CAD build for the part. Positions are in the model's coordinates, mm. Face numbers are marked on the shaded views. A direction names the side the tool comes from. Give positions to 0.01 mm unless a question says otherwise; leave off trailing zeros. Loops run counter-clockwise (first coordinate to the right, second up) from the corner with the lowest first, then second, coordinate; pieces in that order, holes last. Notation, with made-up numbers: (29.25, 79) -> (82.25, 79) arc R32 ccw to (82.25, 105) -> close; hole circle Ø10 at (6, 89). An arc over 180 degrees is marked (long way). Write each question's results on one line, items separated by ' | '. Start each with the question number.
```python
from build123d import *

# Parameters (mm, degrees)
EXTRUDE_1_DEPTH          = 21
SKETCH_2_R               = 7.5
EXTRUDE_2_DEPTH          = 2
SKETCH_3_R               = 9
EXTRUDE_3_DEPTH          = 3
SKETCH_4_R               = 10
EXTRUDE_4_DEPTH          = 8
SKETCH_5_R               = 7.5
EXTRUDE_5_DEPTH          = 2
CUT_EXTRUDE_1_DEPTH      = 42.106568818
CUT_EXTRUDE_1_DEPTH_BACK = 42.106568818
SKETCH_7_R               = 4
HOLE_WIZARD_G1_21_D      = 19
HOLE_WIZARD_G1_21_DEPTH  = 18
HOLE_WIZARD_G1_21_TIP    = 5.708175881
CHAMFER_1_SIZE           = 1
FILLET_1_R               = 1
SKETCH_10_R              = 5
CUT_EXTRUDE_2_DEPTH      = 40


with BuildPart() as part:
    # Эскиз1 → Бобышка-Вытянуть1 (new body)
    with BuildSketch(Plane(origin=(0, 0, 0), x_dir=(1, 0, 0), z_dir=(0, 1, 0))):
        Polygon((0, 15), (-12.990381057, 7.5), (-12.990381057, -7.5), (0, -15), (12.990381057, -7.5), (12.990381057, 7.5), align=None)
    extrude(amount=EXTRUDE_1_DEPTH)

    # Эскиз2 → Бобышка-Вытянуть2 (add)
    with BuildSketch(Plane(origin=(0, 21, 0), x_dir=(1, 0, 0), z_dir=(0, 1, 0))):
        with Locations(Location((0, 0, 0), (0, 0, 270))):
            Circle(SKETCH_2_R)
    extrude(amount=EXTRUDE_2_DEPTH)

    # Эскиз3 → Бобышка-Вытянуть3 (add)
    with BuildSketch(Plane(origin=(0, 23, 0), x_dir=(1, 0, 0), z_dir=(0, 1, 0))):
        with Locations(Location((0, 0, 0), (0, 0, 270))):
            Circle(SKETCH_3_R)
    extrude(amount=EXTRUDE_3_DEPTH)

    # Эскиз4 → Бобышка-Вытянуть4 (add)
    with BuildSketch(Plane(origin=(0, 26, 0), x_dir=(1, 0, 0), z_dir=(0, 1, 0))):
        with Locations(Location((0, 0, 0), (0, 0, 270))):
            Circle(SKETCH_4_R)
    extrude(amount=EXTRUDE_4_DEPTH)

    # Эскиз5 → Бобышка-Вытянуть5 (add)
    with BuildSketch(Plane(origin=(0, 34, 0), x_dir=(1, 0, 0), z_dir=(0, 1, 0))):
        with Locations(Location((0, 0, 0), (0, 0, 270))):
            Circle(SKETCH_5_R)
    extrude(amount=EXTRUDE_5_DEPTH)

    # Эскиз6 → Повернуть1 (revolve)
    with BuildSketch(Plane.XY, mode=Mode.PRIVATE) as revolve_1_sk:
        Polygon((-8, 37), (-6, 37), (-6, 36), (-4, 36), (-4, 38), (-8, 38), align=None)
    revolve(revolve_1_sk.sketch.rotate(Axis((0, 36, 0), (0, 1, 0)), 270), axis=Axis((0, 36, 0), (0, 1, 0)))

    # Эскиз7 → Вырез-Вытянуть1 (cut, two sides: drawn at the far end of the back side and taken through both)
    with BuildSketch(Plane(origin=(0, 36, 0), x_dir=(1, 0, 0), z_dir=(0, 1, 0)).offset(-CUT_EXTRUDE_1_DEPTH_BACK)):
        with Locations(Location((0, 0, 0), (0, 0, 90))):
            Circle(SKETCH_7_R)
    extrude(amount=CUT_EXTRUDE_1_DEPTH + CUT_EXTRUDE_1_DEPTH_BACK, mode=Mode.SUBTRACT)

    # Отверстие обработанное метчиком G1/21
    with Locations(Plane(origin=(0, 0, 0), x_dir=(-1, 0, 0), z_dir=(0, -1, 0))):
        with Locations((0, 0)):
            Hole(HOLE_WIZARD_G1_21_D / 2, depth=HOLE_WIZARD_G1_21_DEPTH)
            with Locations((0, 0, -(HOLE_WIZARD_G1_21_DEPTH + HOLE_WIZARD_G1_21_TIP / 2))):  # 118° drill point
                Cone(0, HOLE_WIZARD_G1_21_D / 2, HOLE_WIZARD_G1_21_TIP, mode=Mode.SUBTRACT)

    # Фаска1
    chamfer_1_edges = [part.edges().sort_by_distance(p)[0] for p in [
        (-12.990381057, 21, 0),
        (-6.495190528, 21, 11.25),
        (6.495190528, 21, 11.25),
        (12.990381057, 21, 0),
        (6.495190528, 21, -11.25),
        (-9.5, 0, 0),
        (12.990381057, 0, 0),
        (6.495190528, 0, 11.25),
        (-6.495190528, 0, 11.25),
        (-6.495190528, 21, -11.25),
        (-12.990381057, 0, 0),
        (-6.495190528, 0, -11.25),
        (6.495190528, 0, -11.25),
    ]]
    chamfer(chamfer_1_edges, length=CHAMFER_1_SIZE)

    # Скругление1
    fillet_1_edges = [part.edges().sort_by_distance(p)[0] for p in [
        (12.990381057, 10.5, -7.5),
        (12.990381057, 10.5, 7.5),
        (0, 10.5, 15),
        (-12.990381057, 10.5, 7.5),
        (-12.990381057, 10.5, -7.5),
        (0, 10.5, -15),
    ]]
    fillet(fillet_1_edges, radius=FILLET_1_R)

    # Эскиз10 → Вырез-Вытянуть2 (cut)
    with BuildSketch(Plane(origin=(0, 38, 0), x_dir=(1, 0, 0), z_dir=(0, 1, 0))):
        with Locations(Location((0, 0, 0), (0, 0, 270))):
            Circle(SKETCH_10_R)
    extrude(amount=-CUT_EXTRUDE_2_DEPTH, mode=Mode.SUBTRACT)


solid = part.part
```
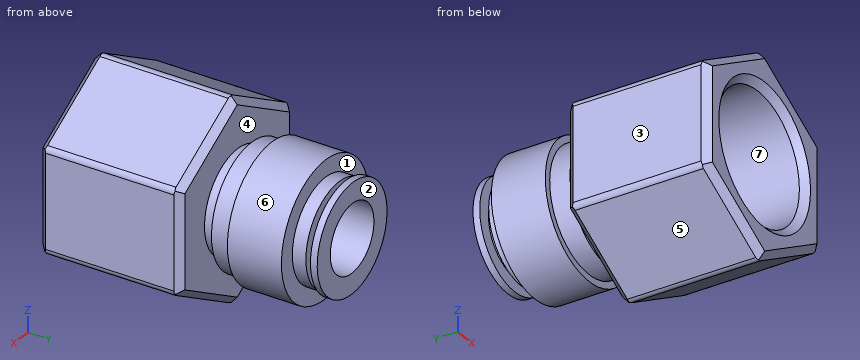
Q1. Saw through at A-A, the plane y = 5. List the corners of the cut face in (x, z).
Q2. Mould opens along Y. For the marked faces 1, 2 and 3 say: pulls with the +Y half, pulls with the -Y half, needs draft (parallel to the pull), parting line crosses it, or undercut.
Q3. Saw through at C-C, the plane x = 11.25. List the corners of the cut face in (y, z), then the cut area to 3 significant figures.
Q4. Drop flat-ended pins along their axis: pin 1 (5.5 mm diameter, centred on x = 3, z = -4, fed in from -Y); pin 2 (6 mm diameter, centred on x = 0, z = 0, fed in from -Y); pin 3 (5 mm diameter, centred on x = -2.5, z = 1.5, fed in from -Y); pin 4 (1.5 mm diameter, centred on x = -6.5, z = 0.5, fed in from -Y). Give the stop position or say it passes through.
Q5. Saw through at B-B, the plane z = 12. List the corners of the cut face in (x, y).
Q6. Saw through at D-D, the plane y = 33.5. List the corners of the cut face in (x, z).
Q7. Which spindle directions (+Z, -Z, +X, -X, +Y, -Y) get a long thin tool onto all of the face, cutting with end or side? Do the marked faces 4, 5, 6 and 7. Say none if no direction does.
Q8. Wall check: L1, parallel to Z at x = 0, y = 11.5; L2, parallel to X at y = 14.5, z = 0; L3, parallel to X at y = 30.5, z = 0. Give the ranges that are in metal, low to high.
Answer block:
1) outline: (-12.99, -6.92) arc R1 ccw to (-12.49, -7.79) -> (-0.5, -14.71) arc R1 ccw to (0.5, -14.71) -> (12.49, -7.79) arc R1 ccw to (12.99, -6.92) -> (12.99, 6.92) arc R1 ccw to (12.49, 7.79) -> (0.5, 14.71) arc R1 ccw to (-0.5, 14.71) -> (-12.49, 7.79) arc R1 ccw to (-12.99, 6.92) -> close; hole circle Ø19 at (0, 0)
2) face 1: undercut | face 2: pulls with the +Y half | face 3: needs draft
3) outline: (0, -7.35) -> (1, -8.5) -> (20, -8.5) -> (21, -7.35) -> (21, 7.35) -> (20, 8.5) -> (1, 8.5) -> (0, 7.35) -> close | area: 355 mm2
4) pin 1: stops at y = 19.05 | pin 2: passes through | pin 3: stops at y = 20.45 | pin 4: stops at y = 19.34
5) outline: (-5.2, 1) -> (-3.2, 0) -> (3.2, 0) -> (5.2, 1) -> (5.2, 20) -> (3.2, 21) -> (-3.2, 21) -> (-5.2, 20) -> close
6) outline: circle Ø20 at (0, 0); hole circle Ø10 at (0, 0)
7) face 4: none | face 5: -Z, -X, +Y, -Y | face 6: +Y | face 7: -Y
8) L1: z = -14.85 to -9.5, 9.5 to 14.85 | L2: x = -12.99 to -9.5, 9.5 to 12.99 | L3: x = -10 to -5, 5 to 10
